Model file for the job. Use its own axes, mm. A direction names the side the tool comes from. Coordinates: 2 decimals unless noted, no trailing zeros. Write each loop counter-clockwise with the first axis right and the second up, starting at its lowest first coordinate (ties: lowest second). Pieces come first, ordered by that corner, then holes.
Q1. Drill centre lines: probe 1 along Y at (x, z) = (20, 38); probe 2 along Z at (x, y) = (58.5, 55); probe 3 along Y at (x, z) = (110, 7.5). Where is each one in solid material? Low to high.
Q2. Pull direction Y, two halves, no side cores. Call faces 5 (the flat face through (51, 46, 7.938)), 6 (the cylindrical face through (133.345, 46.105, 3.913)), 7 (the cylindrical face through (59.54, 70.08, 3.91)), 8 (the cylindrical face through (27.95, 91.49, 73.02)): released by +Y, released by -Y, zero draft, split by the parting line, or undercut.
Q3. Band-saw the part on A-A, the plane z = 24. Write the cut outline in (x, y), plus the area to 3 significant figures.
Q4. Band-saw the part on C-C, the plane z = 41.5. Write the cut outline in (x, y), plus the area to 3 significant figures.
Q5. Band-saw the part on D-D, the plane y = 16. Write the cut outline in (x, z).
Q6. Band-saw the part on B-B, the plane x = 70. Write the cut outline in (y, z).
Q7. Pin check, flat tips, straight feed: P1, Ø16.5, axis at y = 84.5, z = 21.5, coming from the +X side; P2, Ø12, axis at y = 24, z = 8.5, coming from the -X side; P3, Ø25, axis at x = 91.5, y = 39, coming from the +Z side; P4, Ø6.5, axis at x = 90.5, z = 5.5, coming from the -Y side. Stop position of each tip, or through.
Q8. Which spindle directions (+Z, -Z, +X, -X, +Y, -Y) get a long thin tool onto all of the face, cutting with end or side? Do faces 1 (the flat face through (57.15, 2, 17)), 2 (the cylindrical face through (36.449, 91.383, 38.412)), 3 (the flat face through (28, 3.969, 34)), 4 (the flat face through (57.15, 90, 17)). Say none if no direction does.
from build123d import *

# Parameters (mm, degrees)
F0_W     = 57.15
F0_H     = 18.1449148804
F0_R     = 10.3251
F0_H_2   = 16.3959403712
F1_DEPTH = 7.9375
F2_W     = 57.15
F2_H     = 7.9375
F2_R     = 9.92251
F3_DEPTH = 3.96875
F4_W     = 57.15
F4_H     = 7.9375
F4_R     = 9.92251
F5_DEPTH = 3.96875


with BuildPart() as f1:
    # F0 (on Top) → F1 (new body)
    with BuildSketch(Plane.XY):
        with Locations((28.575, 9.0724574402)):
            Rectangle(F0_W, F0_H)
        with BuildLine():
            Line((0, 75.0422115248), (0, 18.1449148804))
            Line((0, 18.1449148804), (57.15, 18.1449148804))
            ThreePointArc((57.15, 18.1449148804), (59.4801290617, 23.0605163329), (64.7604370519, 24.3685632026))
            Line((64.7604370519, 24.3685632026), (111.125, 24.3685632026))
            ThreePointArc((111.125, 24.3685632026), (133.35, 46.5935632026), (111.125, 68.8185632026))
            Line((111.125, 68.8185632026), (64.7604370519, 68.8185632026))
            ThreePointArc((64.7604370519, 68.8185632026), (59.4801290617, 70.1266100723), (57.15, 75.0422115248))
            Line((57.15, 75.0422115248), (0, 75.0422115248))
        make_face()
        with Locations((73.025, 46.5935632026)):
            Circle(F0_R, mode=Mode.SUBTRACT)
        with Locations((111.125, 46.5935632026)):
            Circle(F0_R, mode=Mode.SUBTRACT)
        with Locations((28.575, 83.2401817104)):
            Rectangle(F0_W, F0_H_2)
    extrude(amount=F1_DEPTH)

    # F2 (on face) → F3 (join, symmetric)
    with BuildSketch(Plane.XZ):
        with Locations((28.575, 3.96875)):
            Rectangle(F2_W, F2_H)
        with BuildLine():
            Line((0, 44.45), (0, 7.9375))
            Line((0, 7.9375), (57.15, 7.9375))
            Line((57.15, 7.9375), (57.15, 44.45))
            ThreePointArc((57.15, 44.45), (28.575, 73.025), (0, 44.45))
        make_face()
        with Locations((28.575, 44.45)):
            Circle(F2_R, mode=Mode.SUBTRACT)
    extrude(amount=F3_DEPTH, both=True)

    # F4 (on face) → F5 (join, symmetric)
    with BuildSketch(Plane(origin=(0, 91.438151896, 0), x_dir=(-1, 0, 0), z_dir=(0, 1, 0))):
        with Locations((-28.575, 3.96875)):
            Rectangle(F4_W, F4_H)
        with BuildLine():
            Line((-57.15, 44.45), (-57.15, 7.9375))
            Line((-57.15, 7.9375), (0, 7.9375))
            Line((0, 7.9375), (0, 44.45))
            ThreePointArc((0, 44.45), (-28.575, 73.025), (-57.15, 44.45))
        make_face()
        with Locations((-28.575, 44.45)):
            Circle(F4_R, mode=Mode.SUBTRACT)
    extrude(amount=F5_DEPTH, both=True)


solid = f1.part
Answer sheet:
1. probe 1: y = -3.97 to 3.97, 87.47 to 95.41
1. probe 2: z = 0 to 7.94
1. probe 3: y = 24.37 to 36.33, 56.86 to 68.82
2. face 5: undercut
2. face 6: split by the parting line
2. face 7: released by +Y
2. face 8: zero draft
3. outline: (0, -3.97) - (57.15, -3.97) - (57.15, 3.97) - (0, 3.97) - close; (0, 87.47) - (57.15, 87.47) - (57.15, 95.41) - (0, 95.41) - close
3. area: 907 mm2
4. outline: (0, -3.97) - (19.1, -3.97) - (19.1, 3.97) - (0, 3.97) - close; (0, 87.47) - (19.1, 87.47) - (19.1, 95.41) - (0, 95.41) - close; (38.05, -3.97) - (57.15, -3.97) - (57.15, 3.97) - (38.05, 3.97) - close; (38.05, 87.47) - (57.15, 87.47) - (57.15, 95.41) - (38.05, 95.41) - close
4. area: 606 mm2
5. outline: (0, 0) - (57.15, 0) - (57.15, 7.94) - (0, 7.94) - close
6. outline: (24.37, 0) - (36.72, 0) - (36.72, 7.94) - (24.37, 7.94) - close; (56.47, 0) - (68.82, 0) - (68.82, 7.94) - (56.47, 7.94) - close
7. P1: stops at x = 57.15
7. P2: stops at x = 0
7. P3: stops at z = 7.94
7. P4: stops at y = 24.37
8. face 1: +Z, -Z, +X, -Y
8. face 2: +Y, -Y
8. face 3: +Z, +X, -X
8. face 4: +Z, -Z, +X, +Y
